Build history of the part. All positions in model axes, mm. Face numbers are marked on the shaded views. A direction names the side the tool comes from. Give positions to 0.01 mm unless a question says otherwise; leave off trailing zeros. Order: outer loops, then holes, each group sorted by start corner. A loop starts at its lowest first (then second) coordinate and runs counter-clockwise, first axis right, second up. Notation, with made-up numbers: (69.25, 78.5) - (119.25, 78.5) arc R31 ccw to (119.25, 114.5) - close; hole circle Ø10 at (37, 64). An arc over 180 degrees is marked (long way). Use a Markdown table: item, result.
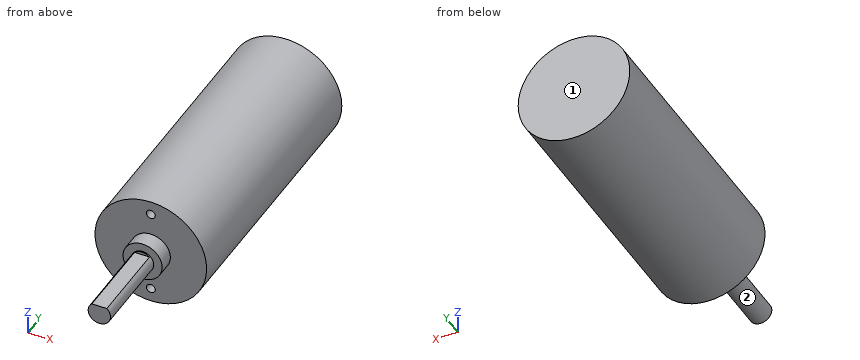
from build123d import *

# Parameters (mm, degrees)
F0_R     = 10
F1_DEPTH = 47.5
F2_R     = 3.5
F3_DEPTH = 2.89
F4_R     = 2
F5_DEPTH = 15.2
F7_D     = 1.6
F7_DEPTH = 6.2
F7_TIP   = 0.4806884952
F9_DEPTH = 15


with BuildPart() as f1:
    # F0 (on Front) → F1 (new body)
    with BuildSketch(Plane.XZ):
        Circle(F0_R)
    extrude(amount=F1_DEPTH)

    # F2 (on face) → F3 (join)
    with BuildSketch(Plane.XZ.offset(47.5)):
        Circle(F2_R)
    extrude(amount=F3_DEPTH)

    # F4 (on face) → F5 (join)
    with BuildSketch(Plane.XZ.offset(50.39)):
        Circle(F4_R)
    extrude(amount=F5_DEPTH)

    # F7
    with Locations(Plane.XZ.offset(47.5)):
        with Locations((0, 7.5), (0, -7.5)):
            Hole(F7_D / 2, depth=F7_DEPTH)
            with Locations((0, 0, -(F7_DEPTH + F7_TIP / 2))):  # 118° drill point
                Cone(0, F7_D / 2, F7_TIP, mode=Mode.SUBTRACT)

    # F8 (on face) → F9 (cut)
    with BuildSketch(Plane.XZ.offset(65.59)):
        with BuildLine():
            ThreePointArc((1.339812841, 1.4848910907), (0, 2), (-1.339812841, 1.4848910907))
            Line((-1.339812841, 1.4848910907), (1.339812841, 1.4848910907))
        make_face()
    extrude(amount=-F9_DEPTH, mode=Mode.SUBTRACT)


solid = f1.part
1) Pin check, flat tips, straight feed: P1, Ø12, axis at y = -57, z = 4.5, coming from the -X side; P2, Ø1, axis at x = -4.5, z = 4, coming from the -Y side; P3, Ø3, axis at y = -47.5, z = -5, coming from the -X side; P4, Ø6, axis at y = -52.5, z = 8, coming from the +X side. Stop position of each tip, or through.
Computed:
| item | result |
|---|---|
| P1 | stops at x = -2 |
| P2 | stops at y = -47.5 |
| P3 | stops at x = -9.37 |
| P4 | passes through |
2) Tool access for the marked faces 1 and 2: list every direction of +Z, -Z, +X, -X, +Y, -Y with a clear straight run to the whole face (end or side of a thin tool).
Computed:
| item | result |
|---|---|
| face 1 | +Z, -Z, +X, -X, +Y |
| face 2 | -Y |
3) Slice it at C-C (x = 7.75). Write the cut outline in (y, z), and give its area (3 significant figures).
Computed:
| item | result |
|---|---|
| outline | (-47.5, -6.32) - (0, -6.32) - (0, 6.32) - (-47.5, 6.32) - close |
| area | 600 mm² |
4) Wall check: line 1 (Z direction, x = 0, y = -43.75); line 2 (Y direction, x = 2.75, z = -7.25); line 3 (X direction, y = -16.5, z = -0.25). Give the ranges that are in metal, low to high. Write a range as from..to.
Computed:
| item | result |
|---|---|
| line 1 | z = -10..-8.3, -6.7..6.7, 8.3..10 |
| line 2 | y = -47.5..0 |
| line 3 | x = -10..10 |
5) Slice it at A-A (z = 0). Write the cut outline in (x, y).
Computed:
| item | result |
|---|---|
| outline | (-10, -47.5) - (-3.5, -47.5) - (-3.5, -50.39) - (-2, -50.39) - (-2, -65.59) - (2, -65.59) - (2, -50.39) - (3.5, -50.39) - (3.5, -47.5) - (10, -47.5) - (10, 0) - (-10, 0) - close |
6) Slice it at D-D (y = -59.5). Write the cut outline in (x, z), and give its area (3 significant figures).
Computed:
| item | result |
|---|---|
| outline | (-1.34, 1.48) arc R2 ccw (long way) to (1.34, 1.48) - close |
| area | 11.6 mm² |
7) Slice it at B-B (y = -16). Write the cut outline in (x, z).
Computed:
| item | result |
|---|---|
| outline | circle Ø20 at (0, 0) |
